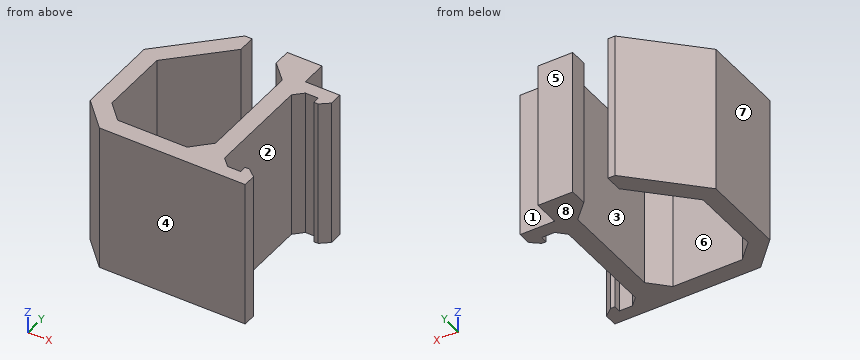
```python
from build123d import *

# Parameters (mm, degrees)
PAD_DEPTH = 17


with BuildPart() as part:
    # Sketch (on XY_Plane of Origin) → Pad (new body)
    with BuildSketch(Plane.XY):
        Polygon((6, 1.52), (6, 2.32), (6.5, 2.32), (7.5, 1.5), (7.5, 0), (-9.3, 0), (-12.434326, 3.228932), (-12.434326, 12.928932), (-5.363258, 20), (-4.534831, 20), (-4.534831, 18), (-10.434326, 12.100505), (-10.434326, 4.021537), (-8.472019, 2), (-0.48, 2), (1.5, 4.021537), (1.5, 16.02), (-0.48, 18), (-0.48, 20), (3.52, 20), (3.52, 17), (7.5, 17), (7.5, 15.5), (6.5, 14.68), (6, 14.68), (6, 15.48), (4.5, 15.48), (3.52, 14.5), (3.52, 2.5), (4.5, 1.52), align=None)
    extrude(amount=-PAD_DEPTH)


solid = part.part
```
Input: part model. Units: mm. Frame: model coordinates. Face numbers are marked on the shaded views. A direction names the side the tool comes from. Give positions to 0.01 mm unless a question says otherwise; leave off trailing zeros. Order: outer loops, then holes, each group sorted by start corner. A loop starts at its lowest first (then second) coordinate and runs counter-clockwise, first axis right, second up. Notation, with made-up numbers: (35, 72.25) - (56, 72.25) arc R21 ccw to (56, 88.25) - close; hole circle Ø6 at (-32, 0). An arc over 180 degrees is marked (long way). One line per item, written item: value.
1. Draft query along X for the marked faces 6, 7 and 8. Return one class per face: released by +X, released by -X, zero draft, split by the parting line, or undercut.
Determined:
face 6: undercut
face 7: released by -X
face 8: zero draft
2. Cut plane A-A, the plane y = 9.75. Output: boundary loops of the cut face in (x, z).
Determined:
outline: (-12.43, -17) - (-10.43, -17) - (-10.43, 0) - (-12.43, 0) - close; (1.5, -17) - (3.52, -17) - (3.52, 0) - (1.5, 0) - close
3. Cut plane D-D, the plane x = -1.25. Output: boundary loops of the cut face in (y, z), and give its area (3 significant figures).
Determined:
outline: (0, -17) - (2, -17) - (2, 0) - (0, 0) - close
area: 34.0 mm2
4. Cut plane B-B, the plane x = 5.5. Output: boundary loops of the cut face in (y, z).
Determined:
outline: (0, -17) - (1.52, -17) - (1.52, 0) - (0, 0) - close; (15.48, -17) - (17, -17) - (17, 0) - (15.48, 0) - close
5. Reachability of the marked faces 1, 2, 3, 4 and 5 from +Z, -Z, +X, -X, +Y, -Y: full face, straight path, thin tool, end or side. Return the list, or none.
Determined:
face 1: +Z, -Z, +X, +Y
face 2: +Z, -Z, +X
face 3: +Z, -Z
face 4: +Z, -Z, +X, -X, -Y
face 5: +Z, -Z, +X, -X, +Y
6. Pin query (flat end, axial travel): pin 1 Ø4 at (y, z) = (8.5, -10.5) entering from +X; pin 2 Ø0.6 at (y, z) = (1.5, -9) entering from -X; pin 3 Ø1.6 at (x, z) = (5.5, -12) entering from +Y. Return the tip coordinate at first contact, or that it passes through.
Determined:
pin 1: x = 3.52
pin 2: x = -11.05
pin 3: y = 17
7. Line query: probe 1 along X at (y, z) = (10.25, -4.75); probe 2 along Y at (x, z) = (6.25, -13); probe 3 along Y at (x, z) = (-4, -4.5). Output: solid intervals per line, ascending.
Determined:
probe 1: -12.43 to -10.43, 1.5 to 3.52
probe 2: 0 to 2.32, 14.68 to 17
probe 3: 0 to 2
